Check sheet for the modelled part. Datum: model origin and axes. Units: mm. Face numbers are marked on the shaded views. A direction names the side the tool comes from. Coordinates: 2 decimals unless noted, no trailing zeros. Write each loop counter-clockwise with the first axis right and the second up, starting at its lowest first coordinate (ties: lowest second). Pieces come first, ordered by that corner, then holes. Notation, with made-up numbers: (53, -11.75) - (108, -11.75) arc R18 cw to (108, 4.25) - close; hole circle Ø3 at (13, -9.75). An arc over 180 degrees is marked (long way). Answer as CSV lines item,"result". Start each with the question number.
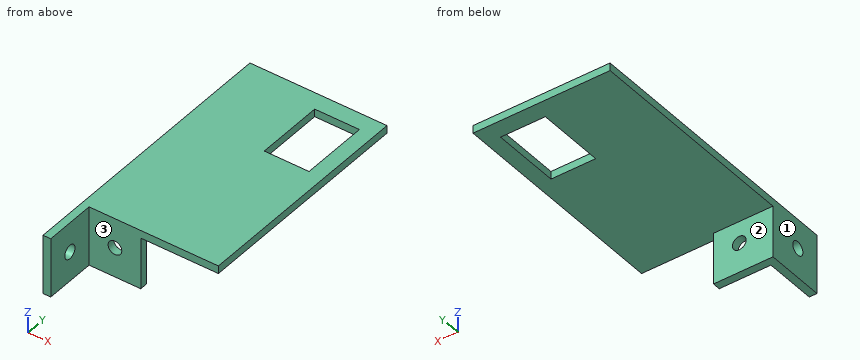
from build123d import *

# Parameters (mm, degrees)
SKETCH_1_W          = 23
SKETCH_1_H          = 23
EXTRUDE_1_DEPTH     = 3
SKETCH_3_R          = 2.65
CUT_EXTRUDE_1_DEPTH = 3
SKETCH_4_W          = 3
SKETCH_4_H          = 23
EXTRUDE_2_DEPTH     = 20
SKETCH_5_R          = 2.65
CUT_EXTRUDE_2_DEPTH = 20
SKETCH_6_W          = 23
SKETCH_6_H          = 3
EXTRUDE_3_DEPTH     = 85
SKETCH_7_W          = 3
SKETCH_7_H          = 88
EXTRUDE_4_DEPTH     = 30
SKETCH_8_W          = 17.3
SKETCH_8_H          = 26.3
CUT_EXTRUDE_3_DEPTH = 20


with BuildPart() as part:
    # 草图1 → 凸台-拉伸1 (new body)
    with BuildSketch(Plane(origin=(0, 0, 0), x_dir=(1, 0, 0), z_dir=(0, 1, 0))):
        with Locations((-3.136363636, -0.122994652)):
            Rectangle(SKETCH_1_W, SKETCH_1_H)
    extrude(amount=EXTRUDE_1_DEPTH)

    # 草图3 → 切除-拉伸1 (cut)
    with BuildSketch(Plane(origin=(0, 3, 0), x_dir=(1, 0, 0), z_dir=(0, 1, 0))):
        with Locations((-1.636363636, -0.122994652)):
            Circle(SKETCH_3_R)
    extrude(amount=-CUT_EXTRUDE_1_DEPTH, mode=Mode.SUBTRACT)

    # 草图4 → 凸台-拉伸2 (add)
    with BuildSketch(Plane.XZ):
        with Locations((-13.136363636, 0.122994652)):
            Rectangle(SKETCH_4_W, SKETCH_4_H)
    extrude(amount=EXTRUDE_2_DEPTH)

    # 草图5 → 切除-拉伸2 (cut)
    with BuildSketch(Plane(origin=(-11.636363636, 0, 0), x_dir=(0, 0, -1), z_dir=(1, 0, 0))):
        with Locations((-0.122994652, -10)):
            Circle(SKETCH_5_R)
    extrude(amount=-CUT_EXTRUDE_2_DEPTH, mode=Mode.SUBTRACT)

    # 草图6 → 凸台-拉伸3 (add)
    with BuildSketch(Plane(origin=(0, 3, 0), x_dir=(1, 0, 0), z_dir=(0, 1, 0))):
        with Locations((-3.136363636, -10.122994652)):
            Rectangle(SKETCH_6_W, SKETCH_6_H)
    extrude(amount=EXTRUDE_3_DEPTH)

    # 草图7 → 凸台-拉伸4 (add)
    with BuildSketch(Plane(origin=(8.363636364, 0, 0), x_dir=(0, 0, -1), z_dir=(1, 0, 0))):
        with Locations((-10.122994652, 44)):
            Rectangle(SKETCH_7_W, SKETCH_7_H)
    extrude(amount=EXTRUDE_4_DEPTH)

    # 草图8 → 切除-拉伸3 (cut)
    with BuildSketch(Plane(origin=(0, 0, 8.622994652), x_dir=(-1, 0, 0), z_dir=(0, 0, -1))):
        with Locations((-24.013636364, 68.15)):
            Rectangle(SKETCH_8_W, SKETCH_8_H)
    extrude(amount=-CUT_EXTRUDE_3_DEPTH, mode=Mode.SUBTRACT)


solid = part.part
(1) Tool access check on the marked faces 1, 2 and 3. Record the directions out of +Z, -Z, +X, -X, +Y, -Y that give a thin tool (end or side, any length) a straight path to the whole face; none if there is none.
(2) Material ranges on probe 1 along X at (y, z) = (-1, 10); probe 2 along Y at (x, z) = (-5, 4.5); probe 3 along Z at (x, y) = (-2.5, 31), recorded low to high. Write a range as from..to.
(3) Cross-section at C-C on z = -9.75. Record the boundary of the cut face in (x, y), plus the area to 3 significant figures.
(4) Cross-section at A-A on y = 69.5. Record the boundary of the cut face in (x, z), plus the area to 3 significant figures.
(5) Cross-section at B-B on z = 1.75. Record the boundary of the cut face in (x, y), plus the area to 3 significant figures.
(6) Go/stop test with flat-tipped pins: P1, Ø2, axis at x = -0.5, z = -8.5, coming from the -Y side; P2, Ø2.5, axis at y = 2, z = -5, coming from the +X side; P3, Ø6, axis at x = 17, y = 45, coming from the -Z side; P4, Ø3, axis at x = -1.64, z = 0.12, coming from the +Y side. Record where each tip stops, or that it passes through.
(7) Cross-section at D-D on y = -10. Record the boundary of the cut face in (x, z), plus the area to 3 significant figures.
Checked values:
1,face 1,"+Z, -Z, -X, +Y, -Y"
1,face 2,"-Z, +X, -X, +Y"
1,face 3,"+Z, -Z, +X, -Y"
2,probe 1,"-14.64..-11.64"
2,probe 2,"0..3"
2,probe 3,"8.62..11.62"
3,outline,"(-14.64, -20) - (-11.64, -20) - (-11.64, 0) - (8.36, 0) - (8.36, 3) - (-14.64, 3) - close"
3,area,"129 mm^2"
4,outline,"(-14.64, 8.62) - (15.36, 8.62) - (15.36, 11.62) - (-14.64, 11.62) - close; (32.66, 8.62) - (38.36, 8.62) - (38.36, 11.62) - (32.66, 11.62) - close"
4,area,"107 mm^2"
5,outline,"(-14.64, -20) - (-11.64, -20) - (-11.64, -12.09) - (-14.64, -12.09) - close; (-14.64, -7.91) - (-11.64, -7.91) - (-11.64, 0) - (-3.73, 0) - (-3.73, 3) - (-14.64, 3) - close; (0.46, 0) - (8.36, 0) - (8.36, 3) - (0.46, 3) - close"
5,area,"104 mm^2"
6,P1,"y = 0"
6,P2,"x = 8.36"
6,P3,"z = 8.62"
6,P4,"through"
7,outline,"(-14.64, -11.38) - (-11.64, -11.38) - (-11.64, -2.53) - (-14.64, -2.53) - close; (-14.64, 2.77) - (-11.64, 2.77) - (-11.64, 11.62) - (-14.64, 11.62) - close"
7,area,"53.1 mm^2"
